Autodesk Inventor part; units mm, degrees
ref_plane "YZ Plane" through (0, 0, 0) normal (1, 0, 0) x (0, 1, 0)
ref_plane "XZ Plane" through (0, 0, 0) normal (0, 1, 0) x (-1, 0, 0)
ref_plane "XY Plane" through (0, 0, 0) normal (0, 0, 1) x (1, 0, 0)
ref_plane "Arbeitsebene1" through (0, 0, 0) normal (0, 0, 1) x (1, 0, 0)
sketch "Skizze1" plane through (0, 0, 0) normal (0, 0, 1) x (1, 0, 0)
  line L0 (159.5, 1) -> (168.5, 1)
  line L1 (159.5, 0) -> (159.5, 1)
  line L2 (161, 0) -> (161, -17)
  line L3 (159.5, 0) -> (161, 0)
  line L4 (168.5, -14) -> (168.5, 1)
  line L5 (159.5, -17) -> (161, -17)
  line L6 (159.5, -17) -> (159.5, -17.5)
  line L7 (161, -19) -> (159.5, -17.5)
  line L8 (168.5, -6) -> (168.5, -38)
  line L9 (168.5, -45) -> (168.5, -30)
  line L10 (168.5, -45) -> (161, -45)
  line L11 (159.5, -22.5) -> (157.9, -22.5) construction
  line L12 (157.9, -22.5) -> (157.9, -40.5) construction
  line L13 (157.9, -40.5) -> (159.5, -40.5) construction
  line L14 (159.5, -40.5) -> (159.5, -22.5) construction
  line L15 (167.9, -24) -> (164, -24) construction
  line L16 (164, -24) -> (164, -39) construction
  line L17 (164, -39) -> (167.9, -39) construction
  line L18 (167.9, -39) -> (167.9, -24) construction
  line L19 (167.9, -25.5) -> (168.5, -25.5) construction
  line L20 (168.5, -25.5) -> (168.5, -37.5) construction
  line L21 (168.5, -37.5) -> (167.9, -37.5) construction
  line L22 (167.9, -37.5) -> (167.9, -25.5) construction
  line L23 (164, -31.5) -> (167.9, -31.5) construction
  line L24 (168.5, -31.5) -> (167.9, -31.5) construction
  line L25 (164, -31.5) -> (159.5, -31.5) construction
  line L26 (159.5, -22.5) -> (160.5261, -23.5261) construction
  line L27 (159.5, -22.5) -> (160.9511, -22.5) construction
  line L28 (164, -31.5) -> (167.9, -31.5) construction
  line L29 (159.5, -22.5) -> (158.7, -21.7) construction
  line L30 (158.7, -21.7) -> (156.9, -23.5) construction
  line L31 (156.9, -23.5) -> (156.9, -19) construction
  line L32 (156.9, -19) -> (161, -19) construction
  line L33 (157.9, -40.5) -> (156.9, -39.5) construction
  line L34 (158.7, -41.3) -> (160.5, -39.5) construction
  line L35 (160.5, -39.5) -> (164, -39.5) construction
  line L36 (164, -39.5) -> (164, -39) construction
  line L37 (160.5261, -23.5261) -> (164, -23.5261) construction
  line L38 (164, -23.5261) -> (164, -24) construction
  line L39 (157.9, -40.5) -> (158.7, -41.3) construction
  line L40 (156.9, -39.5) -> (156.9, -43) construction
  line L41 (161, -45) -> (161, -43)
  line L42 (161, -43) -> (156.9, -43)
  line L43 (161, -19) -> (156.9, -19)
  line L44 (156.9, -19) -> (156.9, -23.5)
  line L45 (156.9, -23.5) -> (158.7, -21.7)
  line L46 (158.7, -21.7) -> (160.5261, -23.5261)
  line L47 (160.5261, -23.5261) -> (164, -23.5261)
  line L48 (164, -23.5261) -> (164, -24)
  line L49 (164, -24) -> (164, -39.5)
  line L50 (164, -39.5) -> (160.5, -39.5)
  line L51 (160.5, -39.5) -> (158.7, -41.3)
  line L52 (158.7, -41.3) -> (156.9, -39.5)
  line L53 (156.9, -39.5) -> (156.9, -43)
  point P0 (0, 0)
  dimension "d0" = 0.6
  dimension "d2" = 6.1
  dimension "d4" = 12
  dimension "d5" = 15
  dimension "d6" = 1.6
  dimension "d7" = 4.5
  dimension "d8" = 18
  dimension "d9" = 45
  dimension "d10" = 1.0261
  dimension "d11" = 6
  dimension "d12" = 1
  dimension "d13" = 0.8
  dimension "d14" = 0.8
  dimension "d15" = 1
  dimension "d16" = 1
  dimension "d17" = 0.8
  dimension "d18" = 1
  dimension "d19" = 2
  dimension "d69" = 3.9
extrude "Extrusion1" add sketch "Skizze1" along normal blind 138.8
sketch "Skizze2" plane through (168.5, -45, 0) normal (1, 0, 0) x (0, 0, -1)
  line L0 (0, 46) -> (-138.8, 46) construction
  line L1 (-69.4, 46) -> (-69.4, 0) construction
  circle A0 centre (4, 23) radius 1.75
  line L2 (0, 15) -> (0, 31)
  line L3 (8, 7) -> (0, 15)
  line L4 (8, 39) -> (8, 7)
  line L5 (0, 31) -> (8, 39)
  circle A1 centre (-142.8, 23) radius 1.75
  line L6 (-138.8, 15) -> (-138.8, 31)
  line L7 (-146.8, 7) -> (-138.8, 15)
  line L8 (-146.8, 39) -> (-146.8, 7)
  line L9 (-138.8, 31) -> (-146.8, 39)
  point P0 (0, 45)
extrude "Extrusion2" add sketch "Skizze2" against normal blind 4.4
sketch "Skizze3" plane through (168.5, 1, 138.8) normal (1, 0, 0) x (0, 0, -1)
  circle A0 centre (142.8, -23) radius 1.75
  circle A1 centre (-4, -23) radius 1.75
  circle A2 centre (142.8, -23) radius 3
  circle A3 centre (-4, -23) radius 3
  point P0 (138.8, -1)
  dimension "d24" = 6
  dimension "d25" = 6
extrude "Extrusion3" cut sketch "Skizze3" against normal blind 3.5
sketch "Skizze4" plane through (156.9, -23.5, 0) normal (-1, 0, 0) x (0, 0, 1)
  line L0 (109.4004, 2.5) -> (119.4004, 2.5)
  line L1 (119.4004, 2.5) -> (119.4004, -2.5)
  line L2 (119.4004, -2.5) -> (109.4004, -2.5)
  line L3 (109.4004, -2.5) -> (109.4004, 2.5)
  line L4 (19.4004, 2.5) -> (29.4004, 2.5)
  line L5 (29.4004, 2.5) -> (29.4004, -2.5)
  line L6 (29.4004, -2.5) -> (19.4004, -2.5)
  line L7 (19.4004, -2.5) -> (19.4004, 2.5)
  point P0 (0, 23.5)
extrude "Extrusion4" add sketch "Skizze4" along normal blind 32.65
chamfer "Fase1" distance 2.5 angle 45 2 edges at (156.9, -26, 114.4004) (156.9, -26, 24.4004)
sketch "Skizze5" plane through (124.25, -26, 29.4004) normal (0, -1, 0) x (1, 0, 0)
  circle A0 centre (5, -5) radius 1.75
  circle A1 centre (5, 85) radius 1.75
  line L0 (32.65, 0) -> (0, 0)
  line L1 (0, -10) -> (0, 0)
  line L2 (0, 80) -> (0, 90)
  line L3 (32.65, 90) -> (0, 90)
  point P0 (-124.25, -29.4004)
  dimension "d33" = 3.5
  dimension "d34" = 3.5
  dimension "d35" = 5
  dimension "d36" = 5
  dimension "d37" = 5
  dimension "d38" = 5
extrude "Extrusion5" cut sketch "Skizze5" against normal blind 36.75
sketch "Skizze7" plane through (156.9, -21, 119.4004) normal (0, 1, 0) x (1, 0, 0)
  circle A0 centre (-27.65, 5) radius 1.75 construction
  circle A1 centre (-27.65, 95) radius 1.75 construction
  line L0 (-29.3243, 7.9) -> (-25.9757, 7.9)
  line L1 (-25.9757, 7.9) -> (-24.3014, 5)
  line L2 (-24.3014, 5) -> (-25.9757, 2.1)
  line L3 (-25.9757, 2.1) -> (-29.3243, 2.1)
  line L4 (-29.3243, 2.1) -> (-30.9986, 5)
  line L5 (-30.9986, 5) -> (-29.3243, 7.9)
  line L6 (-29.3243, 97.9) -> (-25.9757, 97.9)
  line L7 (-25.9757, 97.9) -> (-24.3014, 95)
  line L8 (-24.3014, 95) -> (-25.9757, 92.1)
  line L9 (-25.9757, 92.1) -> (-29.3243, 92.1)
  line L10 (-29.3243, 92.1) -> (-30.9986, 95)
  line L11 (-30.9986, 95) -> (-29.3243, 97.9)
  point P0 (-156.9, 119.4004)
  dimension "d41" = 5.8
  dimension "d43" = 5.8
extrude "Extrusion6" cut sketch "Skizze7" against normal blind 2.5
chamfer "Fase2" distance 2 angle 45 2 edges at (156.9, -21, 114.4004) (156.9, -21, 24.4004)
sketch "Skizze8" plane through (164, -39.5, 0) normal (-1, 0, 0) x (0, 0, 1)
  line L0 (0, 9.5) -> (0, -5.5) construction
  line L1 (0, 0) -> (0, 15.9739) construction
  line L2 (0, 7.987) -> (138.8, 7.987) construction
  line L3 (138.8, -5.5) -> (138.8, 9.5) construction
  circle A0 centre (19.4, 7.987) radius 7.5
  circle A1 centre (39.4, 7.987) radius 7.5
  circle A2 centre (59.4, 7.987) radius 7.5
  circle A3 centre (79.4, 7.987) radius 7.5
  circle A4 centre (99.4, 7.987) radius 7.5
  circle A5 centre (119.4, 7.987) radius 7.5
  point P0 (0, 39.5)
  dimension "d49" = 15
  dimension "d50" = 19.4
  dimension "d53" = 20
  dimension "d58" = 19.4
extrude "Extrusion7" cut sketch "Skizze8" against normal blind 3.9
sketch "Skizze9" plane through (167.9, -31.513, 19.4) normal (-1, 0, 0) x (0, 0, 1)
  circle A0 centre (0, 0) radius 7.5
  circle A1 centre (20, 0) radius 7.5
  circle A2 centre (40, 0) radius 7.5
  circle A3 centre (60, 0) radius 7.5
  circle A4 centre (80, 0) radius 7.5
  circle A5 centre (100, 0) radius 7.5
  circle A6 centre (0, 0) radius 6
  circle A7 centre (20, 0) radius 6
  circle A8 centre (40, 0) radius 6
  circle A9 centre (60, 0) radius 6
  circle A10 centre (80, 0) radius 6
  circle A11 centre (100, 0) radius 6
  point P0 (-19.4, 31.513)
  dimension "d61" = 12
  dimension "d62" = 12
  dimension "d63" = 12
  dimension "d64" = 12
  dimension "d65" = 12
  dimension "d66" = 12
extrude "Extrusion8" cut sketch "Skizze9" against normal blind 3.9 contours A6 | A7 | A8 | A9 | A10 | A11
equation "\"d25\" = d24"
properties part number "TopFrame"
The model under review builds one solid part; all positions refer to its coordinate system, in mm. A direction names the side the tool comes from. Round coordinates to 2 decimals unless told otherwise and drop trailing zeros. Order: outer loops, then holes, each group sorted by start corner. A loop starts at its lowest first (then second) coordinate and runs counter-clockwise, first axis right, second up. Notation, with made-up numbers: (9, 77.25) -> (44, 77.25) arc R15 cw to (44, 88.25) -> close; hole circle Ø11 at (89.5, 67). An arc over 180 degrees is marked (long way). Write item = value, one per line. Start each with the question number.
Item 1: Consider section B-B on z = 142.8. Write out the cut boundary in (x, y).
Item 2: Clearance check with flat-ended pins moving along their axes: pin 1 Ø5 at (y, z) = (-22, -4) entering from -X; pin 2 Ø6 at (x, y) = (139.5, -28.5) entering from -Z; pin 3 Ø12 at (y, z) = (-34.5, 102.5) entering from -X; pin 4 Ø12 at (x, y) = (154.5, -33.5) entering from +Z. State where each tip first meets the part, or that it passes through.
Item 3: Mouldability with a two-part tool opening along Y and no side actions: class faces 1 (the face through (167.9, -26, 76)), 2 (the face through (124.25, -23, 24)), 3 (the face through (166, -34, -4)) as released by +Y, released by -Y, zero draft, split by the parting line, or undercut.
Item 4: Consider section C-C on x = 129. Write out the cut boundary in (y, z).
Item 5: For faces 4 (the face through (140, -26, 114)), 5 (the face through (167.9, -26, 96)), 6 (the face through (166.77, -23.15, 140.03)), list the 3-axis set-ups (+Z, -Z, +X, -X, +Y, -Y) from which the entire face can be reached by the end or side of a thin tool; tool diameter is ignored.
Item 6: For line 1 along Z through (x, y) = (129, -24); line 2 along Y through (x, z) = (168, 19); line 3 along Y through (x, z) = (166.55, 79.4), list the stretches that pass through material, from the lowest coordinate up.
Item 7: Consider section A-A on x = 138. Write out the cut boundary in (y, z).
Conclusion:
q1.outline = (164.1, -34) -> (168.5, -34) -> (168.5, -25) -> (165, -25) -> (165, -23.75) -> (164.1, -23.75) -> close; (164.1, -20.25) -> (165, -20.25) -> (165, -19) -> (168.5, -19) -> (168.5, -10) -> (164.1, -10) -> close
q2.pin_1 = 164.1
q2.pin_2 = 19.4
q2.pin_3 = 156.9
q2.pin_4 = through
q3.face_1 = undercut
q3.face_2 = zero draft
q3.face_3 = released by -Y
q4.outline = (-26, 19.4) -> (-21, 19.4) -> (-21, 21.5) -> (-23.5, 21.5) -> (-23.5, 22.67) -> (-26, 22.67) -> close; (-26, 26.13) -> (-23.5, 26.13) -> (-23.5, 27.3) -> (-21, 27.3) -> (-21, 29.4) -> (-26, 29.4) -> close; (-26, 109.4) -> (-21, 109.4) -> (-21, 111.5) -> (-23.5, 111.5) -> (-23.5, 112.67) -> (-26, 112.67) -> close; (-26, 116.13) -> (-23.5, 116.13) -> (-23.5, 117.3) -> (-21, 117.3) -> (-21, 119.4) -> (-26, 119.4) -> close
q5.face_4 = +Z, -Z, -X, -Y
q5.face_5 = -X
q5.face_6 = +X
q6.line_1 = 19.4 to 22.67, 26.13 to 29.4, 109.4 to 112.67, 116.13 to 119.4
q6.line_2 = -45 to -37.5, -25.53 to 1
q6.line_3 = -45 to -39.01, -24.01 to 1
q7.outline = (-26, 19.4) -> (-21, 19.4) -> (-21, 29.4) -> (-26, 29.4) -> close; (-26, 109.4) -> (-21, 109.4) -> (-21, 119.4) -> (-26, 119.4) -> close
